Part print with two shaded views. Sizes in mm from the minimum x, y, z corner. Round coordinates to 2 decimals unless told otherwise and drop trailing zeros. Write each loop counter-clockwise with the first axis right and the second up, starting at its lowest first coordinate (ties: lowest second). Pieces come first, ordered by that corner, then holes. Notation, with made-up numbers: (47, 67) -> (76, 67) arc R13 ccw to (76, 75) -> close; hole circle Ø5 at (39, 83). An arc over 180 degrees is marked (long way). Answer in a Markdown table with one row per item.
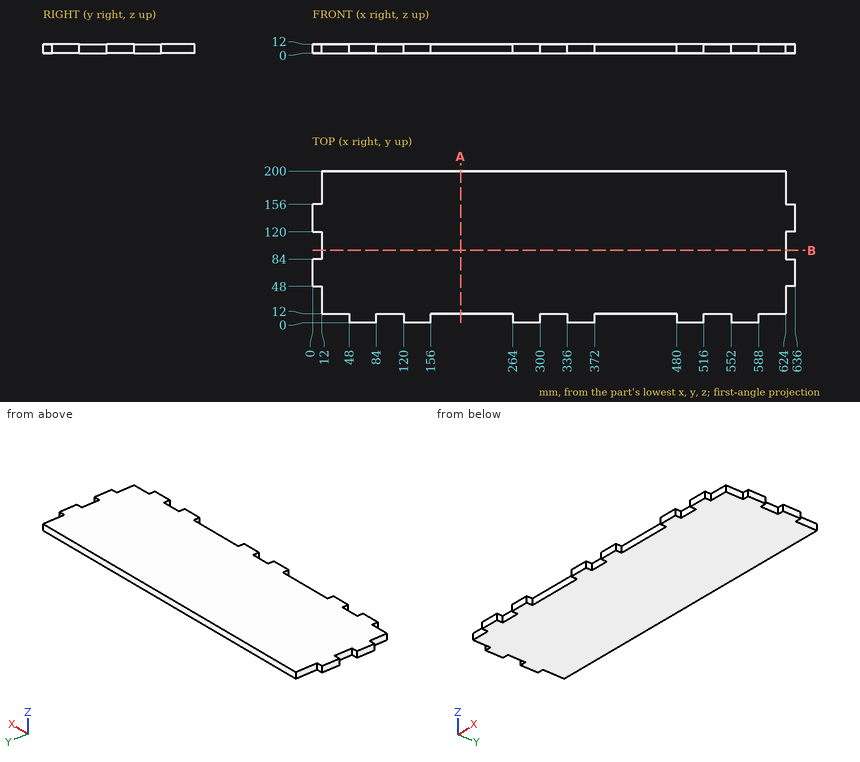
Q1. Wall check: line 1 (X direction, y = 43.5, z = 6.75); line 2 (Y direction, x = 414.5, z = 4.25). Give the ranges that are in metal, low to high. Write a range as [from, to].
A:
| item | result |
|---|---|
| line 1 | [12, 624] |
| line 2 | [12, 200] |
Q2. Saw through at A-A on x = 195. Write the cut outline in (y, z), plus the area to 3 significant figures.
A:
| item | result |
|---|---|
| outline | (12, 0) -> (200, 0) -> (200, 12) -> (12, 12) -> close |
| area | 2,260 mm² |
Q3. Saw through at B-B on y = 95.5. Write the cut outline in (x, z).
A:
| item | result |
|---|---|
| outline | (12, 0) -> (624, 0) -> (624, 12) -> (12, 12) -> close |
Q4. Drop flat-ended pins along their axis: P1, Ø6, axis at y = 181.5, z = 7, coming from the -X side; P2, Ø3.5, axis at x = 8.5, z = 6, coming from the -Y side; P3, Ø3.5, axis at y = 28, z = 7.5, coming from the +X side; P4, Ø3, axis at x = 489, z = 5.5, coming from the -Y side. Give the stop position or say it passes through.
A:
| item | result |
|---|---|
| P1 | x = 12 |
| P2 | y = 48 |
| P3 | x = 624 |
| P4 | y = 0 |
